from build123d import *

# Parameters (mm, degrees)
SKETCH1_R                = 6.9215
BOSS_EXTRUDE1_DEPTH      = 3
SKETCH3_W                = 7
SKETCH3_H                = 4
F_4_0_4_DIAMETER_HOLE1_D = 4
CHAMFER1_SIZE            = 0.1


with BuildPart() as part:
    # Sketch1 → Boss-Extrude1 (new body)
    with BuildSketch(Plane(origin=(1.5, 0, 0), x_dir=(0, 0, -1), z_dir=(1, 0, 0))):
        Circle(SKETCH1_R)
    extrude(amount=-BOSS_EXTRUDE1_DEPTH)

    # Sketch3 → Revolve1 (revolve)
    with BuildSketch(Plane.XY, mode=Mode.PRIVATE) as revolve1_sk:
        with Locations((5, 2)):
            Rectangle(SKETCH3_W, SKETCH3_H)
    revolve(revolve1_sk.sketch.rotate(Axis((1.5, 0, 0), (1, 0, 0)), 270), axis=Axis((1.5, 0, 0), (1, 0, 0)))

    # Ø4.0 (4) Diameter Hole1 (through all)
    with Locations(Plane.ZY.offset(1.5)):
        with Locations((0, 0)):
            Hole(F_4_0_4_DIAMETER_HOLE1_D / 2)

    # Chamfer1
    chamfer1_edges = [part.edges().sort_by_distance(p)[0] for p in [
        (-1.5, 0, 2),
        (8.5, 0, 2),
        (8.5, 0, 4),
    ]]
    chamfer(chamfer1_edges, length=CHAMFER1_SIZE)


solid = part.part
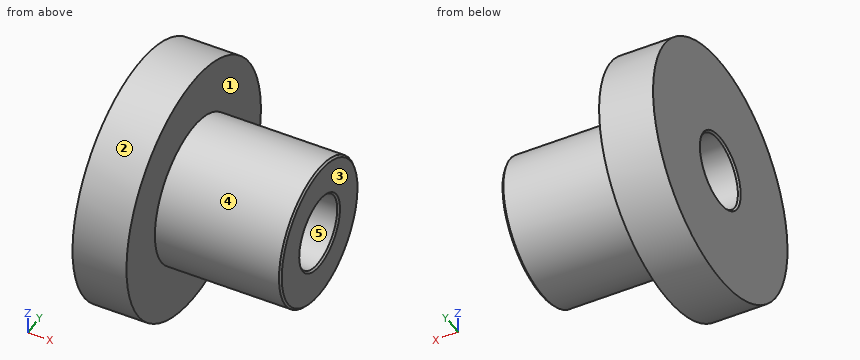
Can you work these out from the model? Positions are in its coordinate system, mm. Face numbers are marked on the shaded views. A direction names the side the tool comes from. Give positions to 0.01 mm unless a question says otherwise; leave off trailing zeros. Order: outer loops, then holes, each group sorted by start corner. A loop starts at its lowest first (then second) coordinate and runs counter-clockwise, first axis right, second up. Notation, with made-up numbers: M 60,44.5 L 92,44.5 A27 cw 92,77.5 Z; hole C 76.5,40.25 d9. An arc over 180 degrees is marked long. Use a Markdown table: item, result. Add a question column.
Item 1: We'd pull the mould along Y, two halves only. Please class the marked faces 3, 4 and 5: +Y half, -Y half, draft (parallel to the pull), parting line (faces both ways), or undercut.
Item 2: For the marked faces 1 and 2, which set-ups out of +Z, -Z, +X, -X, +Y, -Y let a thin tool reach every point of the face, with its end or its side?
Item 3: Suppose I cut it at D-D (x = 1). List the corners of the cut face in (y, z) for me.
Item 4: Will these pins go through, and if not, where does the flat tip stop? pin 1 (3.5 mm diameter, centred on y = 0, z = 0, fed in from +X); pin 2 (4 mm diameter, centred on x = 5.5, y = 2, fed in from +Z); pin 3 (5 mm diameter, centred on x = 0.5, y = -0.5, fed in from +Z); pin 4 (5 mm diameter, centred on x = 2, z = 4, fed in from +Y).
Item 5: If I drill on L1, parallel to Y at x = 3.25, z = 0; L2, parallel to X at y = 2, z = 4.5; L3, parallel to Z at x = 6.75, y = 1, over which ranges is the centre line in solid material (lowest first)? Write a range as [from, to].
Item 6: Suppose I cut it at C-C (x = 6). List the corners of the cut face in (y, z) for me, then the cut area to 3 significant figures.
Item 7: Suppose I cut it at A-A (z = 0). List the corners of the cut face in (x, y) for me, then the cut area to 3 significant figures.
Answer sheet:
| question | item | result |
|---|---|---|
| 1 | face 3 | draft |
| 1 | face 4 | parting line |
| 1 | face 5 | undercut |
| 2 | face 1 | +X |
| 2 | face 2 | +X, -X |
| 3 | outline | C 0,0 d13.84; hole C 0,0 d4 |
| 4 | pin 1 | passes through |
| 4 | pin 2 | stops at z = 4 |
| 4 | pin 3 | stops at z = 6.92 |
| 4 | pin 4 | stops at y = 6.75 |
| 5 | L1 | y = [-4, -2], [2, 4] |
| 5 | L2 | x = [-1.5, 1.5] |
| 5 | L3 | z = [-3.87, -1.73], [1.73, 3.87] |
| 6 | outline | C 0,0 d8; hole C 0,0 d4 |
| 6 | area | 37.7 mm² |
| 7 | outline | M -1.5,-6.92 L 1.5,-6.92 L 1.5,-4 L 8.4,-4 L 8.5,-3.9 L 8.5,-2.1 L 8.4,-2 L -1.4,-2 L -1.5,-2.1 Z; M -1.5,2.1 L -1.4,2 L 8.4,2 L 8.5,2.1 L 8.5,3.9 L 8.4,4 L 1.5,4 L 1.5,6.92 L -1.5,6.92 Z |
| 7 | area | 57.5 mm² |
